from build123d import *

# Parameters (mm, degrees)
F0_W      = 50.8
F0_H      = 50.8
F0_W_2    = 38.1
F0_H_2    = 38.1
F1_DEPTH  = 1206.5
F4_DEPTH  = 603.25
F5_W      = 222.25
F5_H      = 101.6
F6_DEPTH  = 6.35
F7_W      = 6.35
F7_H      = 38.1
F8_DEPTH  = 57.15
F9_R      = 4.7625
F10_DEPTH = 762


with BuildPart() as f1:
    # F0 (on Right) → F1 (new body)
    with BuildSketch(Plane.YZ):
        Rectangle(F0_W, F0_H)
        Rectangle(F0_W_2, F0_H_2, mode=Mode.SUBTRACT)
    extrude(amount=-F1_DEPTH)

    # F3 (on offset) → F4 (join)
    with BuildSketch(Plane.XZ.offset(25.4)):
        Polygon((-876.3, 25.4), (-1079.5, 25.4), (-1079.5, -31.75), (-1073.15, -31.75), (-1073.15, 19.05), (-882.65, 19.05), (-882.65, -31.75), (-876.3, -31.75), align=None)
        Polygon((-127, -31.75), (-127, 25.4), (-330.2, 25.4), (-330.2, -31.75), (-323.85, -31.75), (-323.85, 19.05), (-133.35, 19.05), (-133.35, -31.75), align=None)
    extrude(amount=F4_DEPTH)

    # F5 (on face) → F6 (join)
    with BuildSketch(Plane(origin=(0, 0, -31.75), x_dir=(1, 0, 0), z_dir=(0, 0, -1))):
        with Locations((-228.6, 120.65)):
            Rectangle(F5_W, F5_H)
        with Locations((-228.6, 577.85)):
            Rectangle(F5_W, F5_H)
        with Locations((-977.9, 120.65)):
            Rectangle(F5_W, F5_H)
        with Locations((-977.9, 577.85)):
            Rectangle(F5_W, F5_H)
    extrude(amount=F6_DEPTH)

    # F7 (on face) → F8 (join)
    with BuildSketch(Plane.XY.offset(25.4)):
        with Locations((-231.775, -234.95)):
            Rectangle(F7_W, F7_H)
        with Locations((-987.425, -234.95)):
            Rectangle(F7_W, F7_H)
    extrude(amount=F8_DEPTH)

    # F9 (on face) → F10 (cut)
    with BuildSketch(Plane.YZ.offset(-228.6)):
        with Locations((-234.95, 63.5)):
            Circle(F9_R)
    extrude(amount=-F10_DEPTH, mode=Mode.SUBTRACT)


solid = f1.part
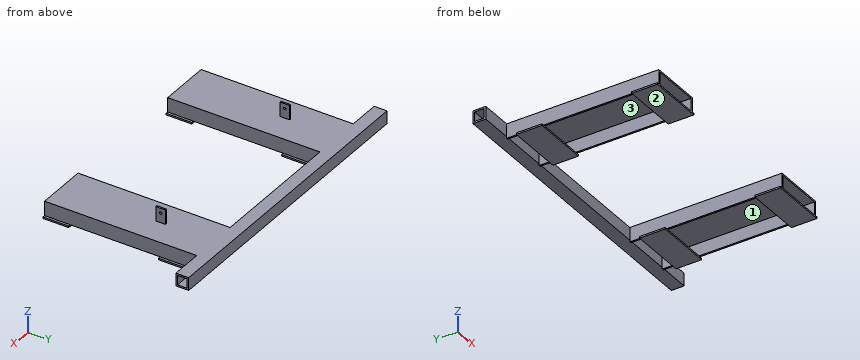
Work out the finished part from the listing and answer in its coordinate system (mm). Face numbers are marked on the shaded views. Give positions to 0.01 mm unless a question says otherwise; leave off trailing zeros. Order: outer loops, then holes, each group sorted by start corner. A loop starts at its lowest first (then second) coordinate and runs counter-clockwise, first axis right, second up. Notation, with made-up numbers: (-24.5, 0) - (0.5, 0) arc R16 cw to (0.5, 27) - close; hole circle Ø9 at (-31.5, 61). An arc over 180 degrees is marked (long way). Answer as CSV lines item,"result". Start each with the question number.
Q1. The part is cut by section B-B (z = -6.5). Write down the section's boundary in (x, y).
Q2. Given pin 1 Ø5 at (x, y) = (-873.5, -143.5) entering from +Z; pin 2 Ø5 at (x, y) = (-131.5, -37) entering from -Z; pin 3 Ø3 at (x, z) = (-129, -28) entering from +Y, each flat-ended and moving along its own axis, determine where each tip first touches the part or whether it passes through.
Q3. Find the intervals of material crossed by L1, parallel to Y at x = -986, z = 63; L2, parallel to X at y = -467, z = -10; L3, parallel to Z at x = -988, y = -234, in increasing order. Write a range as [from, to].
Q4. The part is cut by section C-C (x = -144.5). Write down the section's boundary in (y, z), then the cut area to 3 significant figures.
Q5. The part is cut by section A-A (y = -140). Write down the section's boundary in (x, z) (3 decimals), then the cut area to 3 significant figures.
Q6. The part is cut by section D-D (y = -421). Write down the section's boundary in (x, z).
Q7. The mould has two halves that part along Z. Classify the marked faces 1, 2 and 3: +Z half, -Z half, draft (parallel to the pull), parting line (faces both ways), or undercut.
Check result:
1,outline,"(-1206.5, -25.4) - (-1079.5, -25.4) - (-1079.5, -628.65) - (-1073.15, -628.65) - (-1073.15, -25.4) - (-882.65, -25.4) - (-882.65, -628.65) - (-876.3, -628.65) - (-876.3, -25.4) - (-330.2, -25.4) - (-330.2, -628.65) - (-323.85, -628.65) - (-323.85, -25.4) - (-133.35, -25.4) - (-133.35, -628.65) - (-127, -628.65) - (-127, -25.4) - (0, -25.4) - (0, -19.05) - (-1206.5, -19.05) - close; (-1206.5, 19.05) - (0, 19.05) - (0, 25.4) - (-1206.5, 25.4) - close"
2,pin 1,"stops at z = -31.75"
2,pin 2,"stops at z = -31.75"
2,pin 3,"stops at y = -25.4"
3,L1,"y = [-254, -239.69], [-230.21, -215.9]"
3,L2,"x = [-1079.5, -1073.15], [-882.65, -876.3], [-330.2, -323.85], [-133.35, -127]"
3,L3,"z = [19.05, 58.83], [68.17, 82.55]"
4,outline,"(-628.65, -38.1) - (-527.05, -38.1) - (-527.05, -31.75) - (-628.65, -31.75) - close; (-628.65, 19.05) - (-25.4, 19.05) - (-25.4, -25.4) - (25.4, -25.4) - (25.4, 25.4) - (-628.65, 25.4) - close; (-171.45, -38.1) - (-69.85, -38.1) - (-69.85, -31.75) - (-171.45, -31.75) - close; hole (-19.05, -19.05) - (19.05, -19.05) - (19.05, 19.05) - (-19.05, 19.05) - close"
4,area,"6,250 mm²"
5,outline,"(-1089.025, -38.1) - (-866.775, -38.1) - (-866.775, -31.75) - (-876.3, -31.75) - (-876.3, 25.4) - (-1079.5, 25.4) - (-1079.5, -31.75) - (-1089.025, -31.75) - close; (-339.725, -38.1) - (-117.475, -38.1) - (-117.475, -31.75) - (-127, -31.75) - (-127, 25.4) - (-330.2, 25.4) - (-330.2, -31.75) - (-339.725, -31.75) - close; hole (-1073.15, -31.75) - (-882.65, -31.75) - (-882.65, 19.05) - (-1073.15, 19.05) - close; hole (-323.85, -31.75) - (-133.35, -31.75) - (-133.35, 19.05) - (-323.85, 19.05) - close"
5,area,"6,690 mm²"
6,outline,"(-1079.5, -31.75) - (-1073.15, -31.75) - (-1073.15, 19.05) - (-882.65, 19.05) - (-882.65, -31.75) - (-876.3, -31.75) - (-876.3, 25.4) - (-1079.5, 25.4) - close; (-330.2, -31.75) - (-323.85, -31.75) - (-323.85, 19.05) - (-133.35, 19.05) - (-133.35, -31.75) - (-127, -31.75) - (-127, 25.4) - (-330.2, 25.4) - close"
7,face 1,"undercut"
7,face 2,"-Z half"
7,face 3,"undercut"
